Job drawing, mm, ordinate dimensions from the low corner. One solid piece. A direction names the side the tool comes from. Coordinates: 2 decimals unless noted, no trailing zeros. Loops run counter-clockwise (first coordinate to the right, second up) from the corner with the lowest first, then second, coordinate; pieces in that order, holes last. Notation, with made-up numbers: (-38.75, 4.25) - (14.25, 4.25) arc R26 ccw to (14.25, 26.25) - close; hole circle Ø10 at (66, -7). An arc over 180 degrees is marked (long way). Use a Markdown table: item, result. Add a question column.
1. Drop flat-ended pins along their axis: pin 1 (1 mm diameter, centred on x = 6, z = 4.5, fed in from +Y); pin 2 (8 mm diameter, centred on x = 5.5, y = 5, fed in from -Z); pin 3 (5 mm diameter, centred on x = 11, z = 7.5, fed in from +Y). Give the stop position or say it passes through.
2. 3-axis set-ups, long thin cutter, end or side, ignore diameter. For the marked faces 1, 2 and 3: which of +Z, -Z, +X, -X, +Y, -Y reach the whole face in a straight line?
3. Band-saw the part on A-A, the plane z = 12.5. Give the cut face in (x, y), plus the area to 3 significant figures.
4. Wall check: probe 1 along X at (y, z) = (18, 21.5); probe 2 along Z at (x, y) = (4, 4.5); probe 3 along Z at (x, y) = (11.5, 15.75) (3 decimals). Give the ranges that are in metal, low to high. Write a range as [from, to].
5. Band-saw the part on C-C, the plane x = 10.5. Give the cut face in (y, z), plus the area to 3 significant figures.
6. Band-saw the part on B-B, the plane y = 20. Give the cut face in (x, z).
7. Band-saw the part on D-D, the plane z = 4. Give the cut face in (x, y), plus the area to 3 significant figures.
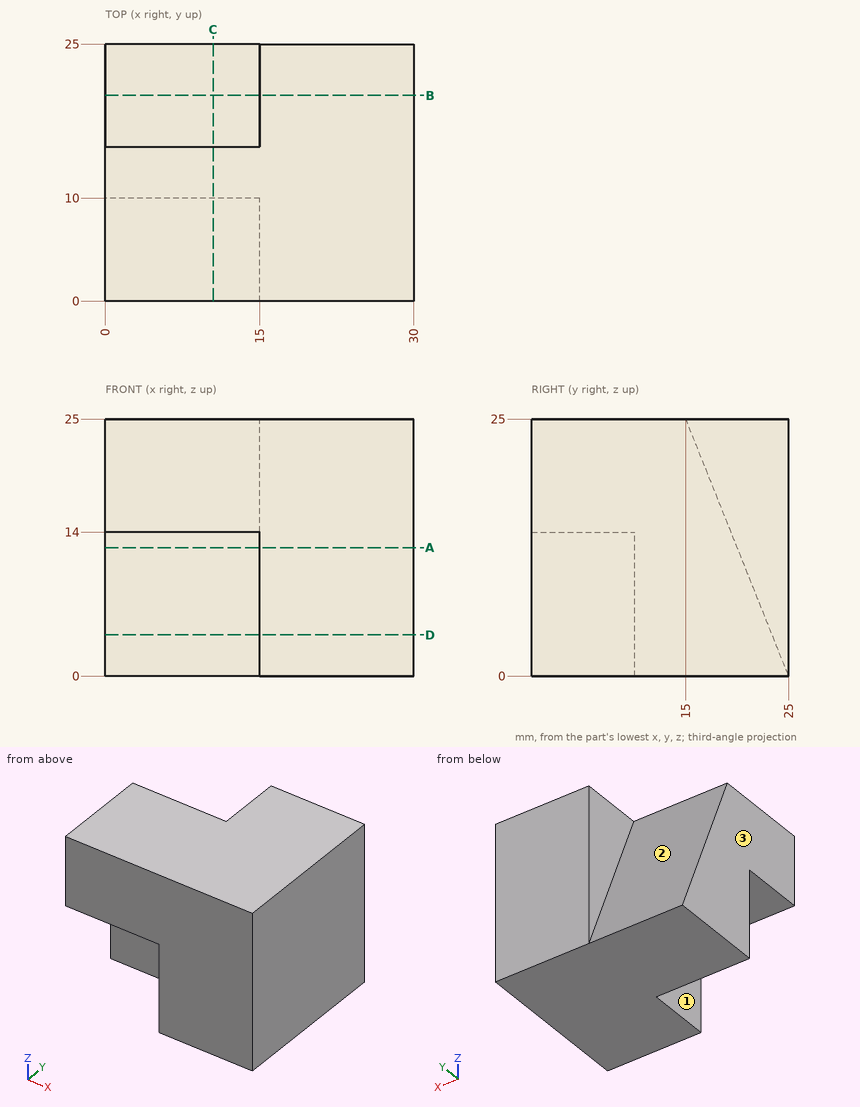
Geometry check:
| question | item | result |
|---|---|---|
| 1 | pin 1 | stops at y = 23.4 |
| 1 | pin 2 | stops at z = 14 |
| 1 | pin 3 | stops at y = 23 |
| 2 | face 1 | -Z, -X, -Y |
| 2 | face 2 | +Z, -X, +Y |
| 2 | face 3 | +Z, -Z, -X, +Y, -Y |
| 3 | outline | (0, 10) - (15, 10) - (15, 0) - (30, 0) - (30, 25) - (15, 25) - (15, 20) - (0, 20) - close |
| 3 | area | 525 mm^2 |
| 4 | probe 1 | x = [15, 30] |
| 4 | probe 2 | z = [14, 25] |
| 4 | probe 3 | z = [0, 23.125] |
| 5 | outline | (0, 14) - (10, 14) - (10, 0) - (25, 0) - (15, 25) - (0, 25) - close |
| 5 | area | 360 mm^2 |
| 6 | outline | (0, 0) - (30, 0) - (30, 25) - (15, 25) - (15, 12.5) - (0, 12.5) - close |
| 7 | outline | (0, 10) - (15, 10) - (15, 0) - (30, 0) - (30, 25) - (15, 25) - (15, 23.4) - (0, 23.4) - close |
| 7 | area | 576 mm^2 |
